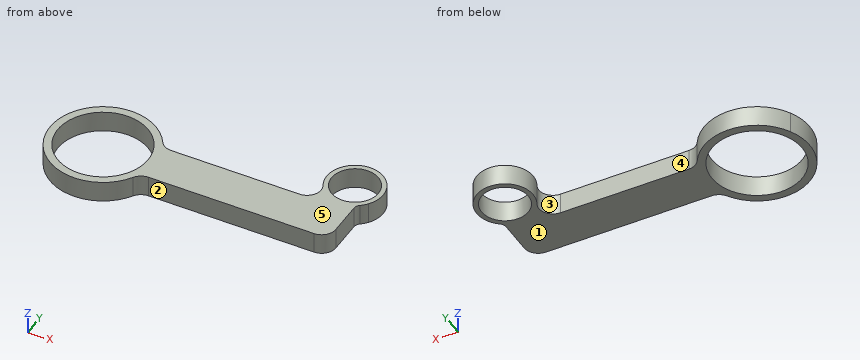
from build123d import *

# Parameters (mm, degrees)
SKETCH1_R           = 40.64
SKETCH1_R_2         = 21.082
BOSS_EXTRUDE1_DEPTH = 19.05


with BuildPart() as part:
    # Sketch1 → Boss-Extrude1 (new body)
    with BuildSketch(Plane.XY):
        with BuildLine():
            Line((-49.036305212, 19.05), (-12.7, 19.05))
            Line((-12.7, 19.05), (66.63309213, 19.05))
            ThreePointArc((66.63309213, 19.05), (77.50872238, 25.1917482), (77.865394753, 37.676666667))
            ThreePointArc((77.865394753, 37.676666667), (86.740959905, 70.989216885), (120.65, 64.77))
            ThreePointArc((120.65, 64.77), (125.73, 49.53), (120.65, 34.29))
            ThreePointArc((120.65, 34.29), (118.290512242, 31.569487758), (115.57, 29.21))
            ThreePointArc((115.57, 29.21), (113.700387337, 26.969806331), (113.03, 24.13))
            Line((113.03, 24.13), (113.03, -6.35))
            ThreePointArc((113.03, -6.35), (109.310256121, -15.330256121), (100.33, -19.05))
            Line((100.33, -19.05), (12.7, -19.05))
            Line((12.7, -19.05), (-49.036305212, -19.05))
            ThreePointArc((-49.036305212, -19.05), (-55.216941357, -20.655418582), (-59.834977799, -25.065789474))
            ThreePointArc((-59.834977799, -25.065789474), (-101.860987289, -47.600385533), (-142.352058824, -22.411764706))
            ThreePointArc((-142.352058824, -22.411764706), (-147.955, 0), (-142.352058824, 22.411764706))
            ThreePointArc((-142.352058824, 22.411764706), (-101.860987289, 47.600385533), (-59.834977799, 25.065789474))
            ThreePointArc((-59.834977799, 25.065789474), (-55.216941357, 20.655418582), (-49.036305212, 19.05))
        make_face()
        with Locations((-100.33, 0)):
            Circle(SKETCH1_R, mode=Mode.SUBTRACT)
        with Locations((100.33, 49.53)):
            Circle(SKETCH1_R_2, mode=Mode.SUBTRACT)
    extrude(amount=BOSS_EXTRUDE1_DEPTH)


solid = part.part
Work out the finished part from the listing and answer in its coordinate system (mm). Face numbers are marked on the shaded views. A direction names the side the tool comes from. Coordinates: 2 decimals unless noted, no trailing zeros. Write each loop counter-clockwise with the first axis right and the second up, starting at its lowest first coordinate (ties: lowest second). Pieces come first, ordered by that corner, then holes. Notation, with made-up numbers: (10.5, 24) - (56.5, 24) arc R16 ccw to (56.5, 36) - close; hole circle Ø4 at (-3.75, 67.5). An arc over 180 degrees is marked (long way). One line per question, with ' | ' between items.
1) Find section D-D, the plane x = -6. Determine the outline of the cut face in (y, z), and give its area (3 significant figures).
Checks:
outline: (-19.05, 0) - (19.05, 0) - (19.05, 19.05) - (-19.05, 19.05) - close | area: 726 mm2
2) Flat-ended cylindrical pins translate along their axes: P1, Ø1.5, axis at x = 42.5, z = 4, coming from the +Y side; P2, Ø1, axis at x = 33, z = 13, coming from the +Y side; P3, Ø8, axis at y = 1, z = 11, coming from the +X side. Find the tip coordinate at first contact, or state that the pin passes through.
Checks:
P1: y = 19.05 | P2: y = 19.05 | P3: x = 113.03
3) For the marked faces 4 and 5, determine the directions among +Z, -Z, +X, -X, +Y, -Y from which every point of the face is accessible in a straight line to the end or side of a thin tool.
Checks:
face 4: +Z, -Z, +Y | face 5: +Z, +X, -X, +Y, -Y
4) The mould has two halves that part along Y. Classify the marked faces 1, 2 and 3: +Y half, -Y half, draft (parallel to the pull), parting line (faces both ways), or undercut.
Checks:
face 1: draft | face 2: -Y half | face 3: undercut
5) Find section C-C, the plane z = 7.75. Determine the outline of the cut face in (x, y) (3 decimals).
Checks:
outline: (-59.835, -25.066) arc R12.7 cw to (-49.036, -19.05) - (100.33, -19.05) arc R12.7 ccw to (113.03, -6.35) - (113.03, 24.13) arc R6.35 cw to (115.57, 29.21) arc R25.4 ccw (long way) to (77.865, 37.677) arc R12.7 cw to (66.633, 19.05) - (-49.036, 19.05) arc R12.7 cw to (-59.835, 25.066) arc R47.625 ccw (long way) to start; hole circle Ø81.28 at (-100.33, 0); hole circle Ø42.164 at (100.33, 49.53)
6) Consider probe 1 along Y at (x, z) = (-100.33, 12) (3 decimals); probe 2 along Y at (x, z) = (100.33, 6); probe 3 along X at (y, z) = (50, 5.5). Determine where each line is inside the solid, lowest interval first. Write a range as [from, to].
Checks:
probe 1: [-47.625, -40.64], [40.64, 47.625] | probe 2: [-19.05, 28.45], [70.61, 74.93] | probe 3: [74.93, 79.25], [121.41, 125.73]
7) Find section A-A, the plane y = 0. Determine the outline of the cut face in (x, z) (3 decimals).
Checks:
outline: (-147.955, 0) - (-140.97, 0) - (-140.97, 19.05) - (-147.955, 19.05) - close; (-59.69, 0) - (113.03, 0) - (113.03, 19.05) - (-59.69, 19.05) - close
8) Find section B-B, the plane x = 96.5. Determine the outline of the cut face in (y, z), and give its area (3 significant figures).
Checks:
outline: (-19.05, 0) - (28.8, 0) - (28.8, 19.05) - (-19.05, 19.05) - close; (70.26, 0) - (74.64, 0) - (74.64, 19.05) - (70.26, 19.05) - close | area: 995 mm2
